Can you work these out from the model? Positions are in its coordinate system, mm. Face numbers are marked on the shaded views. Round coordinates to 2 decimals unless told otherwise and drop trailing zeros. Write each loop counter-clockwise with the first axis right and the second up, starting at its lowest first coordinate (ties: lowest second). Pieces come first, ordered by that corner, then holes.
Q1. If we section it at D-D (x = 81.5): Please give me the cut outline in (y, z), plus the area to 3 significant figures.
Q2. If we section it at B-B (x = 29): Give the number of separate pieces and of enclosed holes in the cut face, plus the area to 3 significant figures.
Q3. Please list where these lines run through material, in increasing order: line 1 along Y through (x, z) = (81.5, 1); line 2 along X through (y, z) = (-75.5, 2.4); line 3 along Y through (x, z) = (5, 1.2).
Q4. We'd pull the mould along Y, two halves only. Please class the marked faces 1 and 2: +Y half, -Y half, draft (parallel to the pull), parting line (faces both ways), or undercut.
Q5. If we section it at A-A (y = 5): Please give me the cut outline in (x, z).
Q6. I'm going to push flat-ended pins straight in: pin 1 Ø3.5 at (x, y) = (29, -71) entering from -Z; pin 2 Ø2.5 at (y, z) = (-40.5, 2.5) entering from -X; pin 3 Ø8 at (x, y) = (69.5, -68.5) entering from +Z. Where does each tip first touch, or does it pass through?
from build123d import *

# Parameters (mm, degrees)
EXTRUDE_2_DEPTH     = 5
SKETCH_3_W          = 30
SKETCH_3_H          = 16.1
CUT_EXTRUDE_1_DEPTH = 2
CUT_EXTRUDE_2_REACH = 155.704
SKETCH_4_R          = 1.55
CUT_EXTRUDE_3_REACH = 155.756
SKETCH_5_W          = 32
SKETCH_5_H          = 56
SKETCH_7_W          = 40.5
SKETCH_7_H          = 40.5
EXTRUDE_4_DEPTH     = 2
SKETCH_8_W          = 30.5
SKETCH_8_H          = 16.5
CUT_EXTRUDE_4_DEPTH = 2
SKETCH_9_R          = 1.55
CUT_EXTRUDE_6_DEPTH = 154.727030805
SKETCH_10_W         = 60
SKETCH_10_H         = 45
EXTRUDE_5_DEPTH     = 2
SKETCH_11_W         = 60
SKETCH_11_H         = 45
CUT_EXTRUDE_8_DEPTH = 2


with BuildPart() as part:
    # 草图1 → 凸台-拉伸2 (new body)
    with BuildSketch(Plane.XY):
        Polygon((0, 0), (0, 30), (120, 30), (120, -96), (0, -96), (0, -56), (45, -56), (45, 0), align=None)
    extrude(amount=EXTRUDE_2_DEPTH)

    # 草图3 → 切除-拉伸1 (cut)
    with BuildSketch(Plane.XY.offset(5)):
        with Locations((17, 10)):
            Rectangle(SKETCH_3_W, SKETCH_3_H)
        with Locations((17, -66)):
            Rectangle(SKETCH_3_W, SKETCH_3_H)
    extrude(amount=-CUT_EXTRUDE_1_DEPTH, mode=Mode.SUBTRACT)

    # 草图4 → 切除-拉伸2 (cut, up to next)
    with BuildSketch(Plane.XY.offset(3), mode=Mode.PRIVATE) as cut_extrude_2_sk1:
        with Locations((29, 15)):
            Circle(SKETCH_4_R)
    cut_extrude_2_tool1 = extrude(cut_extrude_2_sk1.sketch, amount=-CUT_EXTRUDE_2_REACH, mode=Mode.PRIVATE) & part.part
    # 草图4 → 切除-拉伸2 (cut, up to next)
    with BuildSketch(Plane.XY.offset(3), mode=Mode.PRIVATE) as cut_extrude_2_sk2:
        with Locations((29, 5)):
            Circle(SKETCH_4_R)
    cut_extrude_2_tool2 = extrude(cut_extrude_2_sk2.sketch, amount=-CUT_EXTRUDE_2_REACH, mode=Mode.PRIVATE) & part.part
    # 草图4 → 切除-拉伸2 (cut, up to next)
    with BuildSketch(Plane.XY.offset(3), mode=Mode.PRIVATE) as cut_extrude_2_sk3:
        with BuildLine():
            ThreePointArc((5, 16.55), (3.903984489, 16.096015511), (3.45, 15))
            Line((3.45, 15), (5, 15))
            Line((5, 15), (5, 16.55))
        make_face()
    cut_extrude_2_tool3 = extrude(cut_extrude_2_sk3.sketch, amount=-CUT_EXTRUDE_2_REACH, mode=Mode.PRIVATE) & part.part
    # 草图4 → 切除-拉伸2 (cut, up to next)
    with BuildSketch(Plane.XY.offset(3), mode=Mode.PRIVATE) as cut_extrude_2_sk4:
        with BuildLine():
            Line((5, 15), (3.45, 15))
            ThreePointArc((3.45, 15), (5, 13.45), (6.55, 15))
            ThreePointArc((6.55, 15), (6.096015511, 16.096015511), (5, 16.55))
            Line((5, 16.55), (5, 15))
        make_face()
    cut_extrude_2_tool4 = extrude(cut_extrude_2_sk4.sketch, amount=-CUT_EXTRUDE_2_REACH, mode=Mode.PRIVATE) & part.part
    # 草图4 → 切除-拉伸2 (cut, up to next)
    with BuildSketch(Plane.XY.offset(3), mode=Mode.PRIVATE) as cut_extrude_2_sk5:
        with BuildLine():
            ThreePointArc((5, 16.55), (3.903984489, 16.096015511), (3.45, 15))
            Line((3.45, 15), (5, 15))
            Line((5, 15), (5, 16.55))
        make_face()
    cut_extrude_2_tool5 = extrude(cut_extrude_2_sk5.sketch, amount=-CUT_EXTRUDE_2_REACH, mode=Mode.PRIVATE) & part.part
    # 草图4 → 切除-拉伸2 (cut, up to next)
    with BuildSketch(Plane.XY.offset(3), mode=Mode.PRIVATE) as cut_extrude_2_sk6:
        with BuildLine():
            Line((5, 15), (3.45, 15))
            ThreePointArc((3.45, 15), (5, 13.45), (6.55, 15))
            ThreePointArc((6.55, 15), (6.096015511, 16.096015511), (5, 16.55))
            Line((5, 16.55), (5, 15))
        make_face()
    cut_extrude_2_tool6 = extrude(cut_extrude_2_sk6.sketch, amount=-CUT_EXTRUDE_2_REACH, mode=Mode.PRIVATE) & part.part
    # 草图4 → 切除-拉伸2 (cut, up to next)
    with BuildSketch(Plane.XY.offset(3), mode=Mode.PRIVATE) as cut_extrude_2_sk7:
        with Locations((5, 5)):
            Circle(SKETCH_4_R)
    cut_extrude_2_tool7 = extrude(cut_extrude_2_sk7.sketch, amount=-CUT_EXTRUDE_2_REACH, mode=Mode.PRIVATE) & part.part
    # 草图4 → 切除-拉伸2 (cut, up to next)
    with BuildSketch(Plane.XY.offset(3), mode=Mode.PRIVATE) as cut_extrude_2_sk8:
        with Locations((5, -61)):
            Circle(SKETCH_4_R)
    cut_extrude_2_tool8 = extrude(cut_extrude_2_sk8.sketch, amount=-CUT_EXTRUDE_2_REACH, mode=Mode.PRIVATE) & part.part
    # 草图4 → 切除-拉伸2 (cut, up to next)
    with BuildSketch(Plane.XY.offset(3), mode=Mode.PRIVATE) as cut_extrude_2_sk9:
        with Locations((5, -71)):
            Circle(SKETCH_4_R)
    cut_extrude_2_tool9 = extrude(cut_extrude_2_sk9.sketch, amount=-CUT_EXTRUDE_2_REACH, mode=Mode.PRIVATE) & part.part
    # 草图4 → 切除-拉伸2 (cut, up to next)
    with BuildSketch(Plane.XY.offset(3), mode=Mode.PRIVATE) as cut_extrude_2_sk10:
        with Locations((29, -61)):
            Circle(SKETCH_4_R)
    cut_extrude_2_tool10 = extrude(cut_extrude_2_sk10.sketch, amount=-CUT_EXTRUDE_2_REACH, mode=Mode.PRIVATE) & part.part
    # 草图4 → 切除-拉伸2 (cut, up to next)
    with BuildSketch(Plane.XY.offset(3), mode=Mode.PRIVATE) as cut_extrude_2_sk11:
        with Locations((29, -71)):
            Circle(SKETCH_4_R)
    cut_extrude_2_tool11 = extrude(cut_extrude_2_sk11.sketch, amount=-CUT_EXTRUDE_2_REACH, mode=Mode.PRIVATE) & part.part
    add(cut_extrude_2_tool1.solids().sort_by_distance((29, 15, 3))[0], mode=Mode.SUBTRACT)
    add(cut_extrude_2_tool2.solids().sort_by_distance((29, 5, 3))[0], mode=Mode.SUBTRACT)
    add(cut_extrude_2_tool3.solids().sort_by_distance((4.34216, 15.65784, 3))[0], mode=Mode.SUBTRACT)
    add(cut_extrude_2_tool4.solids().sort_by_distance((5.21928, 14.78072, 3))[0], mode=Mode.SUBTRACT)
    add(cut_extrude_2_tool5.solids().sort_by_distance((4.34216, 15.65784, 3))[0], mode=Mode.SUBTRACT)
    add(cut_extrude_2_tool6.solids().sort_by_distance((5.21928, 14.78072, 3))[0], mode=Mode.SUBTRACT)
    add(cut_extrude_2_tool7.solids().sort_by_distance((5, 5, 3))[0], mode=Mode.SUBTRACT)
    add(cut_extrude_2_tool8.solids().sort_by_distance((5, -61, 3))[0], mode=Mode.SUBTRACT)
    add(cut_extrude_2_tool9.solids().sort_by_distance((5, -71, 3))[0], mode=Mode.SUBTRACT)
    add(cut_extrude_2_tool10.solids().sort_by_distance((29, -61, 3))[0], mode=Mode.SUBTRACT)
    add(cut_extrude_2_tool11.solids().sort_by_distance((29, -71, 3))[0], mode=Mode.SUBTRACT)

    # 草图5 → 切除-拉伸3 (cut, up to next)
    with BuildSketch(Plane.XY.offset(5), mode=Mode.PRIVATE) as cut_extrude_3_sk1:
        with Locations((33, -28)):
            Rectangle(SKETCH_5_W, SKETCH_5_H)
    cut_extrude_3_tool1 = extrude(cut_extrude_3_sk1.sketch, amount=-CUT_EXTRUDE_3_REACH, mode=Mode.PRIVATE) & part.part
    add(cut_extrude_3_tool1.solids().sort_by_distance((33, -28, 5))[0], mode=Mode.SUBTRACT)

    # 草图7 → 凸台-拉伸4 (add)
    with BuildSketch(Plane.XY.offset(5)):
        with Locations((79.25, -35.75)):
            Rectangle(SKETCH_7_W, SKETCH_7_H)
    extrude(amount=EXTRUDE_4_DEPTH)

    # 草图8 → 切除-拉伸4 (cut)
    with BuildSketch(Plane.XY.offset(5)):
        with Locations((69.5, -70.5)):
            Rectangle(SKETCH_8_W, SKETCH_8_H)
    extrude(amount=-CUT_EXTRUDE_4_DEPTH, mode=Mode.SUBTRACT)

    # 草图9 → 切除-拉伸6 (cut, through all)
    with BuildSketch(Plane.XY.offset(3)):
        with Locations((81.5, -65.5)):
            Circle(SKETCH_9_R)
        with Locations((57.5, -65.5)):
            Circle(SKETCH_9_R)
        with Locations(Location((57.5, -75.5, 0), (0, 0, 180))):
            Circle(SKETCH_9_R)
        with Locations((81.5, -75.5)):
            Circle(SKETCH_9_R)
    extrude(amount=-CUT_EXTRUDE_6_DEPTH, mode=Mode.SUBTRACT)

    # 草图10 → 凸台-拉伸5 (add)
    with BuildSketch(Plane.XY.offset(7)):
        with Locations((89, -33.5)):
            Rectangle(SKETCH_10_W, SKETCH_10_H)
    extrude(amount=-EXTRUDE_5_DEPTH)

    # 草图11 → 切除-拉伸8 (cut)
    with BuildSketch(Plane.XY.offset(5)):
        with Locations((89, -33.5)):
            Rectangle(SKETCH_11_W, SKETCH_11_H)
    extrude(amount=CUT_EXTRUDE_8_DEPTH, mode=Mode.SUBTRACT)


solid = part.part
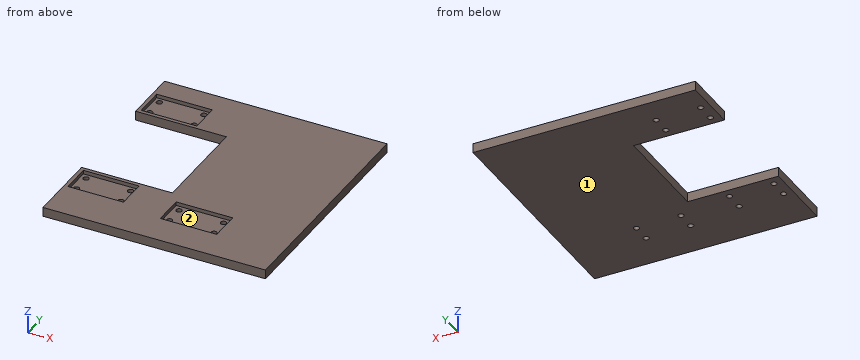
A:
1. outline: (-96, 0) - (-77.05, 0) - (-77.05, 3) - (-78.75, 3) - (-78.75, 5) - (-96, 5) - close; (-73.95, 0) - (-67.05, 0) - (-67.05, 3) - (-73.95, 3) - close; (-63.95, 0) - (30, 0) - (30, 5) - (-62.25, 5) - (-62.25, 3) - (-63.95, 3) - close
1. area: 578 mm2
2. separate pieces: 6
2. enclosed holes: 0
2. area: 248 mm2
3. line 1: y = -96 to -77.05, -73.95 to -67.05, -63.95 to 30
3. line 2: x = 0 to 55.95, 59.05 to 79.95, 83.05 to 120
3. line 3: y = -96 to -72.55, -69.45 to -62.55, -59.45 to -56, 0 to 3.45, 6.55 to 13.45, 16.55 to 30
4. face 1: draft
4. face 2: undercut
5. outline: (0, 0) - (3.45, 0) - (3.45, 3) - (2, 3) - (2, 5) - (0, 5) - close; (6.55, 0) - (27.45, 0) - (27.45, 3) - (6.55, 3) - close; (30.55, 0) - (120, 0) - (120, 5) - (32, 5) - (32, 3) - (30.55, 3) - close
6. pin 1: stops at z = 0
6. pin 2: stops at x = 49
6. pin 3: stops at z = 3
